Check sheet for the modelled part. Datum: model origin and axes. Units: mm. A direction names the side the tool comes from. Round coordinates to 2 decimals unless told otherwise and drop trailing zeros. Loops run counter-clockwise (first coordinate to the right, second up) from the corner with the lowest first, then second, coordinate; pieces in that order, holes last. Notation, with made-up numbers: M 25,89 L 45,89 A22 ccw 45,101 Z; hole C -10.75,-26 d8. An arc over 180 degrees is marked long. One line per question, with ' | ' between items. Start each with the question number.
(1) Thickness scan on probe 1 along Y at (x, z) = (0, 8.9); probe 2 along Y at (x, z) = (-0.25, 2); probe 3 along Z at (x, y) = (-2, -1.75). Record the ranges inside material, lowest first. Write a range as [from, to].
(2) Section check A-A (z = 4.25). Record the boundary of the cut face in (x, y) (3 decimals).
(3) Section check D-D (z = 9.5). Record the boundary of the cut face in (x, y).
(4) Go/stop test with flat-tipped pins: P1, Ø1.9, axis at x = 0.5, z = 4.5, coming from the +Y side; P2, Ø4, axis at x = -2.5, z = 1.5, coming from the -Y side; P3, Ø1.9, axis at x = -1, y = 1, coming from the -Z side; P4, Ø1.5, axis at x = 2.5, z = 4, coming from the -Y side. Record where each tip stops, or that it passes through.
(5) Section check B-B (x = 0). Record the boundary of the cut face in (y, z).
(6) Tool access check on faces 1 (the face through (-3, 2, 0)), 2 (the face through (-1.9, -0.08, 9.48)). Record the directions out of +Z, -Z, +X, -X, +Y, -Y that give a thin tool (end or side, any length) a straight path to the whole face; none if there is none.
(7) Section check C-C (y = 1.5). Record the boundary of the cut face in (x, z), and give its area (3 significant figures).
(8) Draft check along X on faces 3 (the face through (2.826, -1.601, 3.944)), 4 (the face through (0, 0, 12)), 5 (the face through (-5.158, 3.955, 5.916)). Enter one of: +X half, -X half, draft (parallel to the pull), parting line (faces both ways), or undercut.
Autodesk Fusion 360 part; units mm, degrees
sketch "post void" plane through (0, 0, 0) normal (0, 0, 1) x (1, 0, 0)
  circle A0 centre (0, 0) radius 3.75
  line L0 (0, 0) -> (1.875, 3.2476)
  line L1 (0, 0) -> (3.75, 0) construction
  line L2 (0, 0) -> (-1.875, 3.2476)
  line L3 (0, 0) -> (-3.75, 0)
  line L4 (0, 0) -> (-1.875, -3.2476)
  line L5 (0, 0) -> (1.875, -3.2476)
  line L6 (0, 0) -> (3.75, 0)
  line L7 (3.75, 0) -> (1.875, -3.2476)
  line L8 (1.875, -3.2476) -> (-1.875, -3.2476)
  line L9 (-1.875, -3.2476) -> (-3.75, 0)
  line L10 (-3.75, 0) -> (-1.875, 3.2476)
  line L11 (-1.875, 3.2476) -> (1.875, 3.2476)
  line L12 (1.875, 3.2476) -> (3.75, 0)
  dimension "d32" = 7.5
  dimension "d34" = 60
  dimension "d35" = 3.75
  dimension "d36" = 60
  dimension "d37" = 3.75
  dimension "d38" = 60
  dimension "d39" = 3.75
  dimension "d40" = 60
  dimension "d41" = 3.75
  dimension "d42" = 60
  dimension "d43" = 3.75
  dimension "d44" = 60
  dimension "d45" = 3.75
sketch "Wall" plane through (0, 0, 0) normal (0, 0, 1) x (1, 0, 0)
  circle A0 centre (0, 0) radius 6.5
  dimension "d46" = 13
extrude "Extrude1" add sketch "Wall" along normal blind 12
extrude "Extrude2" cut sketch "post void" along normal blind 8 contours L5 L6 L7 | L0 L6 L12 | L0 L2 L11 | L4 L5 L8 | L2 L3 L10 | L3 L4 L9
sketch "Sketch3" plane through (0, 0, 0) normal (0, 0, 1) x (1, 0, 0)
  circle A0 centre (0, 0) radius 1.9
  dimension "d51" = 3.8
extrude "Extrude3" cut sketch "Sketch3" along normal blind 11
equation "d35 = ( 7.5 / 2 ) * 1 mm"
equation "d37 = ( 7.5 / 2 ) * 1 mm"
equation "d39 = ( 7.5 / 2 ) * 1 mm"
equation "d41 = ( 7.5 / 2 ) * 1 mm"
equation "d43 = ( 7.5 / 2 ) * 1 mm"
equation "d45 = ( 7.5 / 2 ) * 1 mm"
equation "d49 = 10.00 mm - 2 mm"
The answers:
1) probe 1: [-6.5, -1.9], [1.9, 6.5] | probe 2: [-6.5, -3.25], [3.25, 6.5] | probe 3: [8, 12]
2) outline: C 0,0 d13; hole M -3.75,0 L -1.875,-3.248 L 1.875,-3.248 L 3.75,0 L 1.875,3.248 L -1.875,3.248 Z
3) outline: C 0,0 d13; hole C 0,0 d3.8
4) P1: y = 6.5 | P2: y = -6.48 | P3: z = 8 | P4: y = -6.26
5) outline: M -6.5,0 L -3.25,0 L -3.25,8 L -1.9,8 L -1.9,11 L 1.9,11 L 1.9,8 L 3.25,8 L 3.25,0 L 6.5,0 L 6.5,12 L -6.5,12 Z
6) face 1: -Z, +X, -X, +Y, -Y | face 2: -Z
7) outline: M -6.32,0 L -2.88,0 L -2.88,8 L -1.17,8 L -1.17,11 L 1.17,11 L 1.17,8 L 2.88,8 L 2.88,0 L 6.32,0 L 6.32,12 L -6.32,12 Z | area: 98.6 mm²
8) face 3: undercut | face 4: draft | face 5: parting line
